For this review, take the finished solid that the model builds, in its own axes (mm). Round coordinates to 2 decimals unless told otherwise and drop trailing zeros. Loops run counter-clockwise (first coordinate to the right, second up) from the corner with the lowest first, then second, coordinate; pieces in that order, holes last.
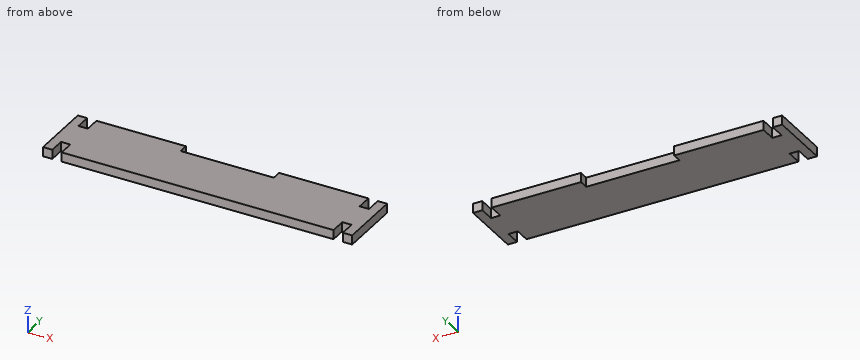
```python
from build123d import *

# Parameters (mm, degrees)
SKETCH1_W            = 199
SKETCH1_H            = 40
BOSS_EXTRUDE1_DEPTH  = 6
SKETCH2_W            = 6
SKETCH2_H            = 10
CUT_EXTRUDE1_DEPTH   = 204.068953806
LPATTERN1_COUNT      = 2
LPATTERN1_PITCH      = 181
LPATTERN1_COUNT_DIR2 = 2
LPATTERN1_PITCH_DIR2 = 30
SKETCH3_W            = 60
SKETCH3_H            = 6
CUT_EXTRUDE2_DEPTH   = 204.068953806


with BuildPart() as part:
    # Sketch1 → Boss-Extrude1 (new body)
    with BuildSketch(Plane.XY):
        with Locations((-99.5, 20)):
            Rectangle(SKETCH1_W, SKETCH1_H)
    extrude(amount=BOSS_EXTRUDE1_DEPTH)

    # Sketch2 → Cut-Extrude1 (cut, through all)
    with BuildSketch(Plane.XY.offset(6)):
        with Locations((-190, 35)):
            Rectangle(SKETCH2_W, SKETCH2_H)
    cut_extrude1 = extrude(amount=-CUT_EXTRUDE1_DEPTH, mode=Mode.SUBTRACT)

    # LPattern1: Cut-Extrude1 2 × 2
    with Locations(*[(i * LPATTERN1_PITCH, -j * LPATTERN1_PITCH_DIR2, 0) for i in range(LPATTERN1_COUNT) for j in range(LPATTERN1_COUNT_DIR2) if (i, j) != (0, 0)]):
        add(cut_extrude1, mode=Mode.SUBTRACT)

    # Sketch3 → Cut-Extrude2 (cut, through all)
    with BuildSketch(Plane.XY.offset(6)):
        with Locations((-99.5, 37)):
            Rectangle(SKETCH3_W, SKETCH3_H)
    extrude(amount=-CUT_EXTRUDE2_DEPTH, mode=Mode.SUBTRACT)


solid = part.part
```
(1) Add section A-A (y = 36.5). Give the boundary of the cut face in (x, z), plus the area to 3 significant figures.
(2) Add section C-C (x = -84). Give the boundary of the cut face in (y, z).
(3) Insertion check: pin 1 Ø12 at (x, y) = (-167.5, 28.5) entering from -Z; pin 2 Ø3 at (x, z) = (-110.5, 3.5) entering from +Y; pin 3 Ø3 at (x, z) = (-10, 3) entering from -Y. Each pin has a flat end and moves straight along its axis. Give the tip position at first contact, or say it passes through.
(4) For L1, parallel to X at y = 32, z = 5.05; L2, parallel to Y at x = -190, z = 3; L3, parallel to Y at x = -97.5, z = 0.8, list the stretches that pass through material, from the lowest coordinate up.
(5) Add section B-B (z = 0.95). Give the boundary of the cut face in (x, y), plus the area to 3 significant figures.
Outcome:
1. outline: (-199, 0) - (-193, 0) - (-193, 6) - (-199, 6) - close; (-187, 0) - (-129.5, 0) - (-129.5, 6) - (-187, 6) - close; (-69.5, 0) - (-12, 0) - (-12, 6) - (-69.5, 6) - close; (-6, 0) - (0, 0) - (0, 6) - (-6, 6) - close
1. area: 762 mm2
2. outline: (0, 0) - (34, 0) - (34, 6) - (0, 6) - close
3. pin 1: stops at z = 0
3. pin 2: stops at y = 34
3. pin 3: stops at y = 10
4. L1: x = -199 to -193, -187 to -12, -6 to 0
4. L2: y = 10 to 30
4. L3: y = 0 to 34
5. outline: (-199, 0) - (-193, 0) - (-193, 10) - (-187, 10) - (-187, 0) - (-12, 0) - (-12, 10) - (-6, 10) - (-6, 0) - (0, 0) - (0, 40) - (-6, 40) - (-6, 30) - (-12, 30) - (-12, 40) - (-69.5, 40) - (-69.5, 34) - (-129.5, 34) - (-129.5, 40) - (-187, 40) - (-187, 30) - (-193, 30) - (-193, 40) - (-199, 40) - close
5. area: 7,360 mm2
